from build123d import *

# Parameters (mm, degrees)
SKETCH1_W           = 42.5
SKETCH1_H           = 11
BOSS_EXTRUDE1_DEPTH = 50
SKETCH2_W           = 82.5
SKETCH2_H           = 4
BOSS_EXTRUDE2_DEPTH = 20
SKETCH3_W           = 82.5
SKETCH3_H           = 4
BOSS_EXTRUDE3_DEPTH = 70
SKETCH4_W           = 10.5
SKETCH4_H           = 34.341245972
SKETCH4_W_2         = 7
BOSS_EXTRUDE4_DEPTH = 42.5
CHAMFER1_SIZE       = 5
SKETCH5_W           = 90
SKETCH5_H           = 82.5
BOSS_EXTRUDE5_DEPTH = 3
SKETCH6_R           = 2.75
CUT_EXTRUDE1_DEPTH  = 118.628081347
SKETCH7_W           = 7.9
SKETCH7_H           = 42.5
SKETCH7_W_2         = 4.4
BOSS_EXTRUDE6_DEPTH = 3
CHAMFER2_SIZE       = 5
CUT_EXTRUDE2_REACH  = 124.45
SKETCH8_W           = 5.5
SKETCH8_H           = 10
SKETCH8_W_2         = 5
SKETCH9_W           = 2
SKETCH9_H           = 10
SKETCH9_W_2         = 5
CUT_EXTRUDE3_DEPTH  = 31.341245972


with BuildPart() as part:
    # Sketch1 → Boss-Extrude1 (new body)
    with BuildSketch(Plane(origin=(0, 0, 0), x_dir=(0, 0, -1), z_dir=(1, 0, 0))):
        with Locations((-46.82408442, -24.747804901)):
            Rectangle(SKETCH1_W, SKETCH1_H)
    extrude(amount=BOSS_EXTRUDE1_DEPTH)

    # Sketch2 → Boss-Extrude2 (add)
    with BuildSketch(Plane.ZY):
        with Locations((46.82408442, -28.247804901)):
            Rectangle(SKETCH2_W, SKETCH2_H)
    extrude(amount=BOSS_EXTRUDE2_DEPTH)

    # Sketch3 → Boss-Extrude3 (add)
    with BuildSketch(Plane(origin=(0, 0, 0), x_dir=(0, 0, -1), z_dir=(1, 0, 0))):
        with Locations((-46.82408442, -28.247804901)):
            Rectangle(SKETCH3_W, SKETCH3_H)
    extrude(amount=BOSS_EXTRUDE3_DEPTH)

    # Sketch4 → Boss-Extrude4 (add)
    with BuildSketch(Plane.XY.offset(68.07408442)):
        with Locations((5.25, -2.077181915)):
            Rectangle(SKETCH4_W, SKETCH4_H)
        with Locations((46.5, -2.077181915)):
            Rectangle(SKETCH4_W_2, SKETCH4_H)
    extrude(amount=-BOSS_EXTRUDE4_DEPTH)

    # Chamfer1
    chamfer1_edges = [part.edges().sort_by_distance(p)[0] for p in [
        (0, -26.247804901, 46.82408442),
        (50, -26.247804901, 46.82408442),
    ]]
    chamfer(chamfer1_edges, length=CHAMFER1_SIZE)

    # Sketch5 → Boss-Extrude5 (add)
    with BuildSketch(Plane.XZ.offset(30.247804901)):
        with Locations((25, 46.82408442)):
            Rectangle(SKETCH5_W, SKETCH5_H)
    extrude(amount=BOSS_EXTRUDE5_DEPTH)

    # Sketch6 → Cut-Extrude1 (cut, through all)
    with BuildSketch(Plane(origin=(0, -19.247804901, 0), x_dir=(1, 0, 0), z_dir=(0, 1, 0))):
        with Locations(Location((25, -36.07408442, 0), (0, 0, 270))):
            Circle(SKETCH6_R)
        with Locations(Location((25, -58.07408442, 0), (0, 0, 270))):
            Circle(SKETCH6_R)
    extrude(amount=-CUT_EXTRUDE1_DEPTH, mode=Mode.SUBTRACT)

    # Sketch7 → Boss-Extrude6 (add)
    with BuildSketch(Plane(origin=(0, -19.247804901, 0), x_dir=(1, 0, 0), z_dir=(0, 1, 0))):
        with Locations((39.05, -46.82408442)):
            Rectangle(SKETCH7_W, SKETCH7_H)
        with Locations((12.7, -46.82408442)):
            Rectangle(SKETCH7_W_2, SKETCH7_H)
    extrude(amount=BOSS_EXTRUDE6_DEPTH)

    # Chamfer2
    chamfer2_edges = [part.edges().sort_by_distance(p)[0] for p in [
        (0, 15.093441071, 46.82408442),
        (50, 15.093441071, 46.82408442),
    ]]
    chamfer(chamfer2_edges, length=CHAMFER2_SIZE)

    # Cut-Extrude2: up to this face of the body (flat: up to its plane)
    cut_extrude2_end = Plane(part.part.faces().sort_by_distance((12.7, -16.247804901, 46.82408442))[0])
    # Sketch8 → Cut-Extrude2 (cut, up to the picked face)
    with BuildSketch(Plane(origin=(0, 15.093441071, 0), x_dir=(1, 0, 0), z_dir=(0, 1, 0)), mode=Mode.PRIVATE) as cut_extrude2_sk1:
        with Locations((7.75, -63.07408442)):
            Rectangle(SKETCH8_W, SKETCH8_H)
    cut_extrude2_tool1 = split(extrude(cut_extrude2_sk1.sketch, amount=-CUT_EXTRUDE2_REACH, mode=Mode.PRIVATE), bisect_by=cut_extrude2_end, keep=Keep.BOTH, mode=Mode.PRIVATE)
    # Sketch8 → Cut-Extrude2 (cut, up to the picked face)
    with BuildSketch(Plane(origin=(0, 15.093441071, 0), x_dir=(1, 0, 0), z_dir=(0, 1, 0)), mode=Mode.PRIVATE) as cut_extrude2_sk2:
        with Locations((47.5, -30.57408442)):
            Rectangle(SKETCH8_W_2, SKETCH8_H)
    cut_extrude2_tool2 = split(extrude(cut_extrude2_sk2.sketch, amount=-CUT_EXTRUDE2_REACH, mode=Mode.PRIVATE), bisect_by=cut_extrude2_end, keep=Keep.BOTH, mode=Mode.PRIVATE)
    add(cut_extrude2_tool1.solids().sort_by(Axis((7.75, 15.093441, 63.074084), (0, -1, 0)))[0], mode=Mode.SUBTRACT)
    add(cut_extrude2_tool2.solids().sort_by(Axis((47.5, 15.093441, 30.574084), (0, -1, 0)))[0], mode=Mode.SUBTRACT)

    # Sketch9 → Cut-Extrude3 (cut)
    with BuildSketch(Plane(origin=(0, 15.093441071, 0), x_dir=(1, 0, 0), z_dir=(0, 1, 0))):
        with Locations((44, -30.57408442)):
            Rectangle(SKETCH9_W, SKETCH9_H)
        with Locations((2.5, -63.07408442)):
            Rectangle(SKETCH9_W_2, SKETCH9_H)
    extrude(amount=-CUT_EXTRUDE3_DEPTH, mode=Mode.SUBTRACT)


solid = part.part
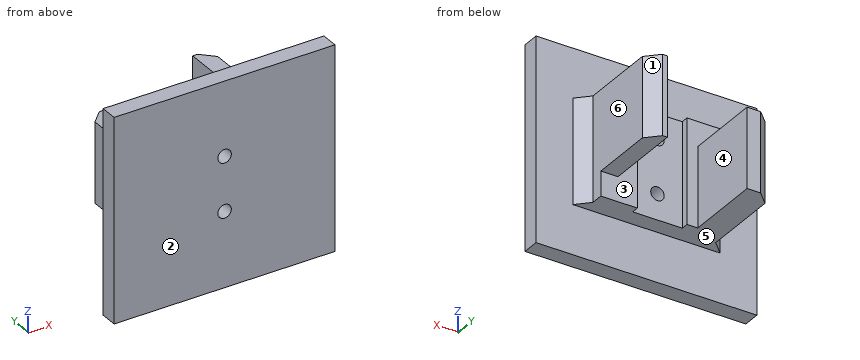
Verification items for the finished model (mm, model axes). Face numbers are marked on the shaded views. A direction names the side the tool comes from. Coordinates: 2 decimals unless noted, no trailing zeros. Loops run counter-clockwise (first coordinate to the right, second up) from the corner with the lowest first, then second, coordinate; pieces in that order, holes last. Notation, with made-up numbers: (22, 3.25) -> (77, 3.25) arc R4 cw to (77, 10.25) -> close; hole circle Ø7 at (37.5, 68). An arc over 180 degrees is marked (long way). Answer as CSV lines item,"result".
1) Cross-section at D-D, the plane x = 13. Record the cut outline in (y, z), then the cut area to 3 significant figures.
Found:
outline,"(-33.25, 5.57) -> (-26.25, 5.57) -> (-26.25, 25.57) -> (-16.25, 25.57) -> (-16.25, 68.07) -> (-26.25, 68.07) -> (-26.25, 88.07) -> (-33.25, 88.07) -> close"
area,"1,000 mm2"
2) Cross-section at B-B, the plane x = 25. Record the cut outline in (y, z).
Found:
outline,"(-33.25, 5.57) -> (-26.25, 5.57) -> (-26.25, 25.57) -> (-19.25, 25.57) -> (-19.25, 33.32) -> (-33.25, 33.32) -> close; (-33.25, 38.82) -> (-19.25, 38.82) -> (-19.25, 55.32) -> (-33.25, 55.32) -> close; (-33.25, 60.82) -> (-19.25, 60.82) -> (-19.25, 68.07) -> (-26.25, 68.07) -> (-26.25, 88.07) -> (-33.25, 88.07) -> close"
3) Release check for a two-part mould opening along X. For the marked faces 1, 2 and 3 record: +X half, -X half, draft (parallel to the pull), parting line (faces both ways), or undercut.
Found:
face 1,"+X half"
face 2,"draft"
face 3,"undercut"
4) Cross-section at C-C, the plane z = 47. Record the cut outline in (x, y).
Found:
outline,"(-20, -33.25) -> (70, -33.25) -> (70, -26.25) -> (55, -26.25) -> (50, -21.25) -> (50, 10.09) -> (45, 15.09) -> (43, 15.09) -> (43, -16.25) -> (35.1, -16.25) -> (35.1, -19.25) -> (14.9, -19.25) -> (14.9, -16.25) -> (10.5, -16.25) -> (10.5, 15.09) -> (5, 15.09) -> (0, 10.09) -> (0, -21.25) -> (-5, -26.25) -> (-20, -26.25) -> close"
5) Thickness scan on L1, parallel to X at y = -3, z = 56; L2, parallel to Y at x = -14, z = 70.5; L3, parallel to Y at x = 12, z = 57. Record the ranges inside material, lowest first. Write a range as from..to.
Found:
L1,"x = 0..10.5, 43..50"
L2,"y = -33.25..-26.25"
L3,"y = -33.25..-16.25"
6) Cross-section at A-A, the plane y = -12.5. Record the cut outline in (x, z).
Found:
outline,"(0, 25.57) -> (10.5, 25.57) -> (10.5, 58.07) -> (0, 58.07) -> close; (43, 35.57) -> (50, 35.57) -> (50, 68.07) -> (43, 68.07) -> close"
7) Depth check by flat-ended pin: pin 1 (16 mm diameter, centred on x = 26, z = 49, fed in from +Y); pin 2 (9.5 mm diameter, centred on y = -11.5, z = 56, fed in from -X); pin 3 (2 mm diameter, centred on y = -15, z = 47, fed in from +X). Enter the tip coordinate at first touch or a pass-through.
Found:
pin 1,"stops at y = -19.25"
pin 2,"stops at x = 0"
pin 3,"stops at x = 50"
8) Tool access check on the marked faces 4, 5 and 6. Record the directions out of +Z, -Z, +X, -X, +Y, -Y that give a thin tool (end or side, any length) a straight path to the whole face; none if there is none.
Found:
face 4,"+Z, -Z, +Y"
face 5,"-Z, +X, -X, +Y"
face 6,"+Z, -Z, +X, +Y"
